Input: dimensioned drawing with shaded views. Units: mm. Origin: part minimum x, y, z. A direction names the side the tool comes from. Round coordinates to 2 decimals unless told otherwise and drop trailing zeros. Write each loop counter-clockwise with the first axis right and the second up, starting at its lowest first coordinate (ties: lowest second). Pieces come first, ordered by that corner, then holes. Notation, with made-up numbers: (59, 47) - (108, 47) arc R23 cw to (108, 65) - close; hole circle Ø11 at (-1.5, 4.5). An arc over 180 degrees is marked (long way). Use one line per item in the form item = value.
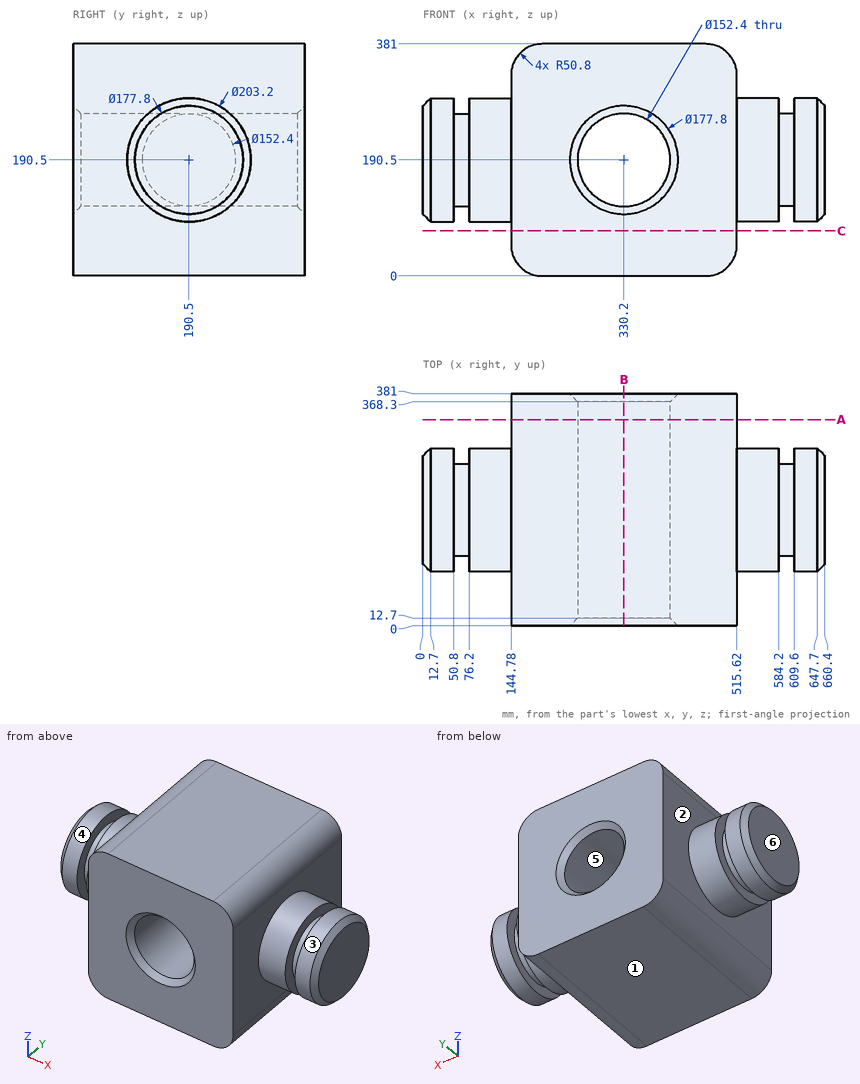
(1) Cut plane A-A on y = 339. Output: boundary loops of the cut face in (x, z), then the cut area to 3 significant figures.
Derived:
outline = (144.78, 50.8) arc R50.8 ccw to (195.58, 0) - (464.82, 0) arc R50.8 ccw to (515.62, 50.8) - (515.62, 330.2) arc R50.8 ccw to (464.82, 381) - (195.58, 381) arc R50.8 ccw to (144.78, 330.2) - close; hole circle Ø152.4 at (330.2, 190.5)
area = 121,000 mm^2
(2) Draft query along X for the marked faces 4, 5 and 6. Return one class per face: released by +X, released by -X, zero draft, split by the parting line, or undercut.
Derived:
face_4 = zero draft
face_5 = undercut
face_6 = released by -X
(3) Material intervals for L1, parallel to Z at x = 330.2, y = 153.5; L2, parallel to X at y = 141, z = 190; L3, parallel to X at y = 135, z = 113.5, sorted ascending.
Derived:
L1 = 0 to 114.3, 266.7 to 381
L2 = 0 to 254, 406.4 to 660.4
L3 = 6.02 to 50.8, 76.2 to 584.2, 609.6 to 654.38
(4) Access query for the marked faces 1, 2 and 3. Directions: +Z, -Z, +X, -X, +Y, -Y. A direction counts if a zero-diameter tool reaches every point of the face in a straight line with its end or side. Return the directions, or none.
Derived:
face_1 = -Z, +X, -X, +Y, -Y
face_2 = -X
face_3 = +X
(5) Cut plane C-C on z = 74. Output: boundary loops of the cut face in (x, y), then the cut area to 3 significant figures.
Derived:
outline = (144.78, 0) - (515.62, 0) - (515.62, 381) - (144.78, 381) - close
area = 141,000 mm^2
(6) First-contact query: pin 1 Ø4 at (x, z) = (539, 144) entering from +Y; pin 2 Ø12 at (x, y) = (588, 255.5) entering from -Z; pin 3 Ø8 at (y, z) = (81.5, 63.5) entering from +X. Flat tips, straight axial feed; report the tip coordinate or a pass-through.
Derived:
pin_1 = 281.84
pin_2 = 108.77
pin_3 = 515.62
(7) Cut plane B-B on x = 330.2. Output: boundary loops of the cut face in (y, z), then the cut area to 3 significant figures.
Derived:
outline = (0, 0) - (381, 0) - (381, 101.6) - (368.3, 114.3) - (12.7, 114.3) - (0, 101.6) - close; (0, 279.4) - (12.7, 266.7) - (368.3, 266.7) - (381, 279.4) - (381, 381) - (0, 381) - close
area = 86,800 mm^2
